Check sheet for the modelled part. Datum: model origin and axes. Units: mm. Give positions to 0.01 mm unless a question says otherwise; leave off trailing zeros. Loops run counter-clockwise (first coordinate to the right, second up) from the corner with the lowest first, then second, coordinate; pieces in that order, holes last. Notation, with made-up numbers: (65.25, 81) - (88.25, 81) arc R31 ccw to (88.25, 107) - close; hole circle Ø1 at (88, 50). An arc over 180 degrees is marked (long way). Answer in a Markdown table with one row per item. Add a question column.
(1) Thickness scan on L1, parallel to X at y = 5.5, z = 0; L2, parallel to Z at x = 200.5, y = 1.5; L3, parallel to X at y = 3.5, z = -0.5. Record the ranges inside material, lowest first.
(2) Sectioned sample at B-B on z = 12. Enter the section's corners in (x, y), then the cut area to 3 significant figures.
(3) Go/stop test with a flat-tipped pin: P1, Ø1, axis at x = 171.5, y = 7, coming from the +Z side (3 decimals). Record where the tip stops, or that it passes through.
(4) Sectioned sample at C-C on x = 101. Enter the section's corners in (y, z) (3 decimals), then the cut area to 4 significant figures.
(5) Sectioned sample at A-A on y = 4.5. Enter the section's corners in (x, z).
(6) Draft check along Z on faces 1 (the face through (215, 5, 0)), 2 (the face through (99, 0, 0)), 3 (the face through (204.957, 4.93, -0.651)). Enter one of: released by +Z, released by -Z, zero draft, split by the parting line, or undercut.
from build123d import *

# Parameters (mm, degrees)
CROQUIS1_R              = 1.5
CROQUIS1_R_2            = 5
SALIENTE_EXTRUIR1_DEPTH = 10


with BuildPart() as part:
    # Croquis1 → Saliente-Extruir1 (new body)
    with BuildSketch(Plane(origin=(0, 0, 0), x_dir=(1, 0, 0), z_dir=(0, 1, 0))):
        with BuildLine():
            Line((0.146382734, 19.996340432), (200, 15))
            ThreePointArc((200, 15), (215, 0), (200, -15))
            Line((200, -15), (0.146382734, -19.996340432))
            ThreePointArc((0.146382734, -19.996340432), (-0.030336377, -19.999196031), (-0.207078355, -19.998927935))
            ThreePointArc((-0.207078355, -19.998927935), (-20, 0), (-0.207078355, 19.998927935))
            ThreePointArc((-0.207078355, 19.998927935), (-0.030336377, 19.999196031), (0.146382734, 19.996340432))
        make_face()
        with Locations(Location((7.5, 0, 0), (0, 0, 270))):
            Circle(CROQUIS1_R, mode=Mode.SUBTRACT)
        with Locations(Location((3.75, -6.495190528, 0), (0, 0, 270))):
            Circle(CROQUIS1_R, mode=Mode.SUBTRACT)
        with Locations(Location((-3.75, -6.495190528, 0), (0, 0, 270))):
            Circle(CROQUIS1_R, mode=Mode.SUBTRACT)
        with Locations(Location((-7.5, 0, 0), (0, 0, 270))):
            Circle(CROQUIS1_R, mode=Mode.SUBTRACT)
        with Locations(Location((-3.75, 6.495190528, 0), (0, 0, 270))):
            Circle(CROQUIS1_R, mode=Mode.SUBTRACT)
        with Locations(Location((3.75, 6.495190528, 0), (0, 0, 270))):
            Circle(CROQUIS1_R, mode=Mode.SUBTRACT)
        with Locations(Location((200, 0, 0), (0, 0, 270))):
            Circle(CROQUIS1_R_2, mode=Mode.SUBTRACT)
    extrude(amount=SALIENTE_EXTRUIR1_DEPTH)


solid = part.part
Reply:
| question | item | result |
|---|---|---|
| 1 | L1 | -20 to -9, -6 to 6, 9 to 195, 205 to 215 |
| 1 | L2 | -14.99 to -4.97, 4.97 to 14.99 |
| 1 | L3 | -19.99 to -8.91, -6.09 to 6.09, 8.91 to 195.03, 204.97 to 214.99 |
| 2 | outline | (-16, 0) - (209, 0) - (209, 10) - (-16, 10) - close |
| 2 | area | 2,250 mm^2 |
| 3 | P1 | z = 15.725 |
| 4 | outline | (0, -17.475) - (10, -17.475) - (10, 17.475) - (0, 17.475) - close |
| 4 | area | 349.5 mm^2 |
| 5 | outline | (-0.21, -20) arc R10 ccw to (0.15, -20) - (200, -15) arc R15 ccw to (200, 15) - (0.15, 20) arc R10 ccw to (-0.21, 20) arc R20 ccw to start; hole circle Ø3 at (-7.5, 0); hole circle Ø3 at (-3.75, -6.5); hole circle Ø3 at (-3.75, 6.5); hole circle Ø3 at (3.75, -6.5); hole circle Ø3 at (3.75, 6.5); hole circle Ø3 at (7.5, 0); hole circle Ø10 at (200, 0) |
| 6 | face 1 | split by the parting line |
| 6 | face 2 | zero draft |
| 6 | face 3 | undercut |
